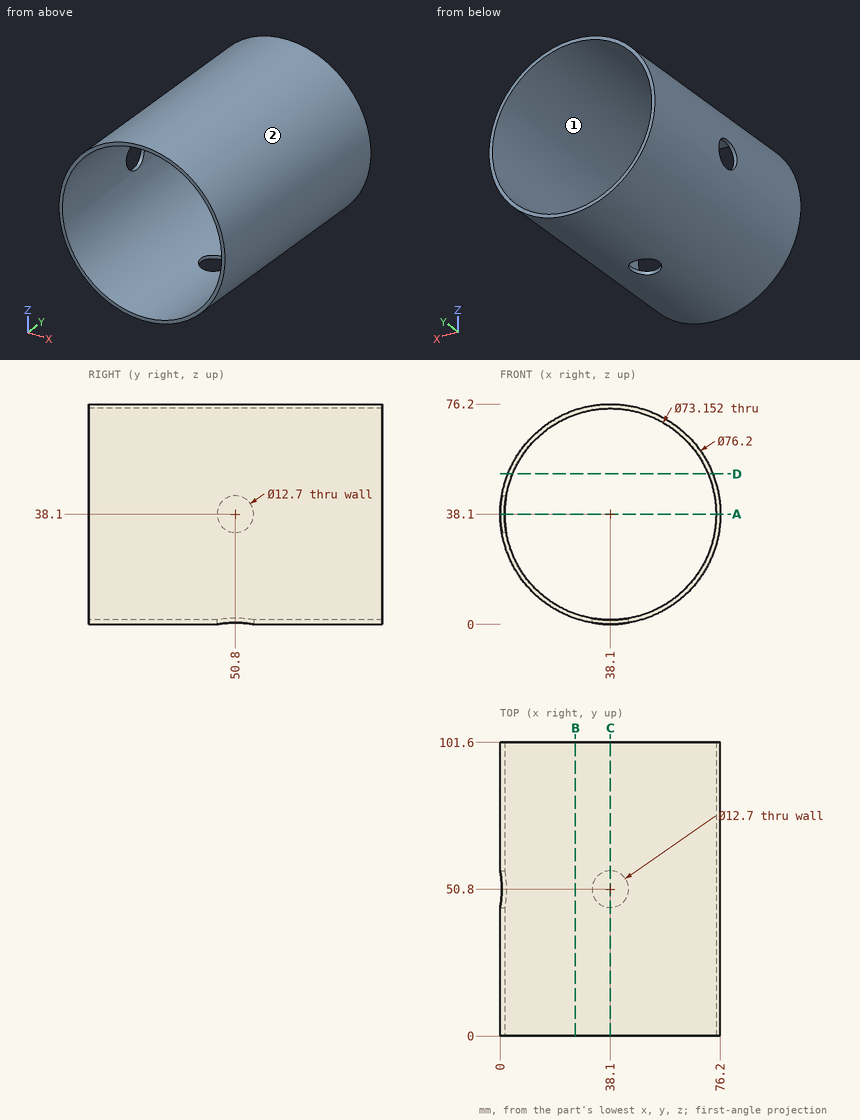
Print and shaded views of the part. All mm, measured from the part's lowest x, y and z. Give positions to 0.01 mm unless a question says otherwise; leave off trailing zeros. Loops run counter-clockwise (first coordinate to the right, second up) from the corner with the lowest first, then second, coordinate; pieces in that order, holes last. Notation, with made-up numbers: (-22, 29) -> (-5, 29) arc R22 cw to (-5, 61) -> close; hole circle Ø3 at (-39, -0.5). An arc over 180 degrees is marked (long way). Use CSV: the item, a comma, the result in double quotes. Start each with the question number.
1) Flat gauge pins, fed straight in: pin 1 Ø10 at (x, y) = (49.5, 10.5) entering from -Z; pin 2 Ø10 at (y, z) = (89, 38) entering from +X; pin 3 Ø5 at (x, y) = (53.5, 89) entering from +Z; pin 4 Ø8 at (x, z) = (68, 14) entering from -Y. Where does each tip first touch, or does it go through?
2) Slice it at C-C on x = 38.1. Give the cut face in (y, z).
3) Slice it at D-D on z = 52. Give the cut face in (x, y).
4) Slice it at A-A on z = 38.1. Give the cut face in (x, y).
5) Slice it at B-B on x = 26. Give the cut face in (y, z), plus the area to 3 significant figures.
6) Mould opens along Z. For the marked faces 1 and 2 say: released by +Z, released by -Z, zero draft, split by the parting line, or undercut.
7) Wall check: line 1 (Z direction, x = 38, y = 39.5); line 2 (X direction, y = 57, z = 38.1). Give the ranges that are in metal, low to high.
Computed values:
1,pin 1,"stops at z = 0.54"
1,pin 2,"stops at x = 76.2"
1,pin 3,"stops at z = 73.95"
1,pin 4,"stops at y = 0"
2,outline,"(0, 0) -> (44.45, 0) -> (44.45, 1.52) -> (0, 1.52) -> close; (0, 74.68) -> (101.6, 74.68) -> (101.6, 76.2) -> (0, 76.2) -> close; (57.15, 0) -> (101.6, 0) -> (101.6, 1.52) -> (57.15, 1.52) -> close"
3,outline,"(2.63, 0) -> (4.27, 0) -> (4.27, 101.6) -> (2.63, 101.6) -> close; (71.93, 0) -> (73.57, 0) -> (73.57, 101.6) -> (71.93, 101.6) -> close"
4,outline,"(0, 0) -> (1.52, 0) -> (1.52, 44.45) -> (0, 44.45) -> close; (0, 57.15) -> (1.52, 57.15) -> (1.52, 101.6) -> (0, 101.6) -> close; (74.68, 0) -> (76.2, 0) -> (76.2, 101.6) -> (74.68, 101.6) -> close"
5,outline,"(0, 1.97) -> (101.6, 1.97) -> (101.6, 3.58) -> (0, 3.58) -> close; (0, 72.62) -> (101.6, 72.62) -> (101.6, 74.23) -> (0, 74.23) -> close"
5,area,"327 mm^2"
6,face 1,"undercut"
6,face 2,"split by the parting line"
7,line 1,"z = 0 to 1.52, 74.68 to 76.2"
7,line 2,"x = 74.68 to 76.2"
